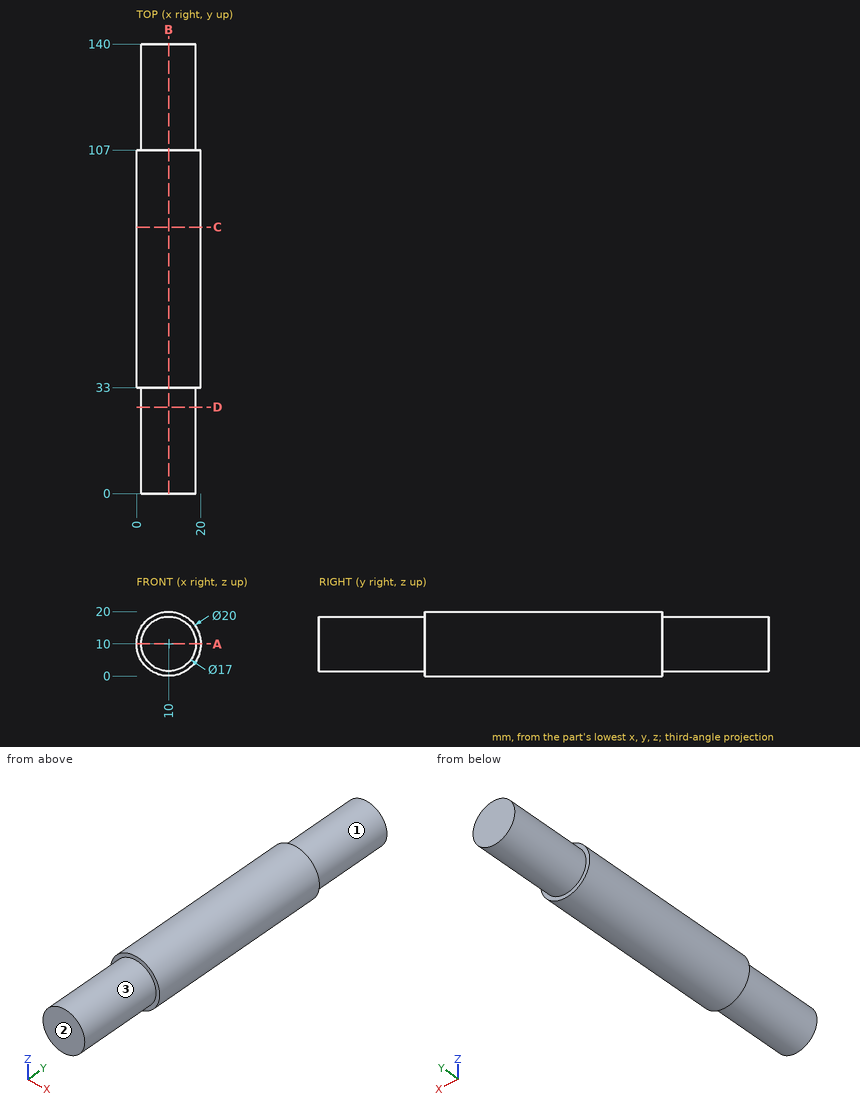
Study the drawing (mm; zero at the part's minimum x, y, z) and answer. A direction names the side the tool comes from. Give positions to 0.01 mm unless a question says otherwise; leave off trailing zeros. Loops run counter-clockwise (first coordinate to the right, second up) from the corner with the lowest first, then second, coordinate; pieces in that order, holes last. Notation, with made-up numbers: (23, -3.5) -> (76, -3.5) arc R34 ccw to (76, 34.5) -> close; hole circle Ø4 at (27, 53.25). An arc over 180 degrees is marked (long way). Write item = value, one per line. Start each with the question number.
(1) Find the intervals of material crossed by probe 1 along Z at (x, y) = (10, 22); probe 2 along Y at (x, z) = (19, 8); probe 3 along X at (y, z) = (37.5, 9.25), in increasing order. Write a range as from..to.
(2) Find section A-A on z = 10. Give the vertices of the cut face in (x, y), and give its area (3 significant figures).
(3) Find section B-B on x = 10. Give the vertices of the cut face in (y, z), and give its area (3 significant figures).
(4) Which of the six approach directions +Z, -Z, +X, -X, +Y, -Y give full straight-line access (tool end or side, diameter ignored) to the marked faces 1, 2 and 3?
(5) Find section C-C on y = 83. Give the vertices of the cut face in (x, z), and give its area (3 significant figures).
(6) Find section D-D on y = 27. Give the vertices of the cut face in (x, z), and give its area (3 significant figures).
(7) Given pin 1 Ø3 at (y, z) = (75.5, 15.5) entering from -X; pin 2 Ø6 at (x, y) = (13.5, 108.5) entering from +Z; pin 3 Ø1.5 at (x, y) = (15.5, 87.5) entering from +Z, each flat-ended and moving along its own axis, determine where each tip first touches the part or whether it passes through.
From the geometry:
q1.probe_1 = 1.5..18.5
q1.probe_2 = 33..107
q1.probe_3 = 0.03..19.97
q2.outline = (0, 33) -> (1.5, 33) -> (1.5, 0) -> (18.5, 0) -> (18.5, 33) -> (20, 33) -> (20, 107) -> (18.5, 107) -> (18.5, 140) -> (1.5, 140) -> (1.5, 107) -> (0, 107) -> close
q2.area = 2,600 mm^2
q3.outline = (0, 1.5) -> (33, 1.5) -> (33, 0) -> (107, 0) -> (107, 1.5) -> (140, 1.5) -> (140, 18.5) -> (107, 18.5) -> (107, 20) -> (33, 20) -> (33, 18.5) -> (0, 18.5) -> close
q3.area = 2,600 mm^2
q4.face_1 = +Y
q4.face_2 = +Z, -Z, +X, -X, -Y
q4.face_3 = -Y
q5.outline = circle Ø20 at (10, 10)
q5.area = 314 mm^2
q6.outline = circle Ø17 at (10, 10)
q6.area = 227 mm^2
q7.pin_1 = 0.83
q7.pin_2 = 19.96
q7.pin_3 = 18.8
